```python
from build123d import *

# Parameters (mm, degrees)
SKETCH2_W           = 90
SKETCH2_H           = 28
BOSS_EXTRUDE1_DEPTH = 3
SKETCH3_R           = 2.125
SKETCH3_R_2         = 1.075
CUT_EXTRUDE1_DEPTH  = 2
SKETCH5_R           = 1.075
CUT_EXTRUDE3_DEPTH  = 4


with BuildPart() as part:
    # Sketch2 → Boss-Extrude1 (new body)
    with BuildSketch(Plane(origin=(0, 0, 0), x_dir=(1, 0, 0), z_dir=(0, 1, 0))):
        with Locations((10.225806452, 5.983870968)):
            Rectangle(SKETCH2_W, SKETCH2_H)
    extrude(amount=BOSS_EXTRUDE1_DEPTH)

    # Sketch3 → Cut-Extrude1 (cut)
    # profile 1 of 4: a face of its own
    with BuildSketch(Plane(origin=(0, 3, 0), x_dir=(1, 0, 0), z_dir=(0, 1, 0))):
        with Locations(Location((-31.592213033, 16.801890452, 0), (0, 0, 270))):
            Circle(SKETCH3_R)
        with Locations(Location((-31.592213033, 16.801890452, 0), (0, 0, 270))):
            Circle(SKETCH3_R_2, mode=Mode.SUBTRACT)
    # profile 2 of 4: a face of its own
    with BuildSketch(Plane(origin=(0, 3, 0), x_dir=(1, 0, 0), z_dir=(0, 1, 0))):
        with Locations(Location((-31.592213033, -4.834148517, 0), (0, 0, 90))):
            Circle(SKETCH3_R)
        with Locations(Location((-31.592213033, -4.834148517, 0), (0, 0, 90))):
            Circle(SKETCH3_R_2, mode=Mode.SUBTRACT)
    # profile 3 of 4: a face of its own
    with BuildSketch(Plane(origin=(0, 3, 0), x_dir=(1, 0, 0), z_dir=(0, 1, 0))):
        with Locations(Location((52.043825936, -4.834148517, 0), (0, 0, 270))):
            Circle(SKETCH3_R)
        with Locations(Location((52.043825936, -4.834148517, 0), (0, 0, 270))):
            Circle(SKETCH3_R_2, mode=Mode.SUBTRACT)
    # profile 4 of 4: a face of its own
    with BuildSketch(Plane(origin=(0, 3, 0), x_dir=(1, 0, 0), z_dir=(0, 1, 0))):
        with Locations(Location((52.043825936, 16.801890452, 0), (0, 0, 90))):
            Circle(SKETCH3_R)
        with Locations(Location((52.043825936, 16.801890452, 0), (0, 0, 90))):
            Circle(SKETCH3_R_2, mode=Mode.SUBTRACT)
    extrude(amount=-CUT_EXTRUDE1_DEPTH, mode=Mode.SUBTRACT)

    # Sketch5 → Cut-Extrude3 (cut)
    with BuildSketch(Plane(origin=(0, 3, 0), x_dir=(1, 0, 0), z_dir=(0, 1, 0))):
        with Locations(Location((-31.592213033, 16.801890452, 0), (0, 0, 270))):
            Circle(SKETCH5_R)
        with Locations(Location((-31.592213033, -4.834148517, 0), (0, 0, 90))):
            Circle(SKETCH5_R)
        with Locations(Location((52.043825936, -4.834148517, 0), (0, 0, 270))):
            Circle(SKETCH5_R)
        with Locations(Location((52.043825936, 16.801890452, 0), (0, 0, 90))):
            Circle(SKETCH5_R)
    extrude(amount=-CUT_EXTRUDE3_DEPTH, mode=Mode.SUBTRACT)


solid = part.part
```
Design review of the part built by this model. Coordinates are the model's own, in mm. A direction names the side the tool comes from. Give positions to 0.01 mm unless a question says otherwise; leave off trailing zeros. Write each loop counter-clockwise with the first axis right and the second up, starting at its lowest first coordinate (ties: lowest second). Pieces come first, ordered by that corner, then holes.
(1) Wall thickness on line 1 along X through (y, z) = (0.95, -17.5); line 2 along X through (y, z) = (1.4, 6.75): over which ranges is each line inside the solid? List them lowest first.
Checked values:
line 1: x = -34.77 to -32.41, -30.77 to 51.23, 52.86 to 55.23
line 2: x = -34.77 to -32.51, -30.67 to 51.12, 52.96 to 55.23
(2) Tool access review of faces 4 (the face through (49.937, 2.014, -16.525)), 5 (the face through (10, 1, -19.984)): name each direction out of +Z, -Z, +X, -X, +Y, -Y from which nothing blocks a thin tool from reaching the whole face with its end or side.
Checked values:
face 4: +Y
face 5: -Z, +X, -X, +Y, -Y
(3) Clearance check with flat-ended pins moving along their axes: pin 1 Ø3.5 at (x, z) = (51.5, 5.5) entering from +Y; pin 2 Ø2.5 at (x, z) = (52.04, -16.8) entering from +Y. State where each tip first meets the part, or that it passes through.
Checked values:
pin 1: stops at y = 3
pin 2: stops at y = 1
(4) Mouldability with a two-part tool opening along X and no side actions: class faces 1 (the face through (-31.18, 0.51, 3.84)), 2 (the face through (-34.774, 1, -6)), 3 (the face through (10, 3, -6)) as +X half, -X half, draft (parallel to the pull), parting line (faces both ways), or undercut.
Checked values:
face 1: undercut
face 2: -X half
face 3: draft
(5) Add section A-A (y = 1.7). Give the boundary of the cut face in (x, z) (3 decimals).
Checked values:
outline: (-34.774, -19.984) - (55.226, -19.984) - (55.226, 8.016) - (-34.774, 8.016) - close; hole circle Ø4.25 at (-31.592, -16.802); hole circle Ø4.25 at (-31.592, 4.834); hole circle Ø4.25 at (52.044, -16.802); hole circle Ø4.25 at (52.044, 4.834)
